```python
from build123d import *

# Parameters (mm, degrees)
AUFSATZ_LINEAR_START                        = 170
AUFSATZ_LINEAR_AUSTRAGEN2_DEPTH             = 460
SCHNITT_LINEAR_AUSTRAGEN1_REACH             = 14.65
SKIZZE15_R                                  = 4
SCHNITT_LINEAR_AUSTRAGEN1_DIRECTION_2_REACH = 14.65
SKIZZE17_W                                  = 30
SKIZZE17_H                                  = 20
SCHNITT_LINEAR_AUSTRAGEN2_DEPTH             = 12.65
SKIZZE19_W                                  = 17.7
SKIZZE19_H                                  = 170
SCHNITT_LINEAR_AUSTRAGEN3_DEPTH             = 25.15
HOLES_R                                     = 1.5
SCHNITT_LINEAR_AUSTRAGEN5_DEPTH             = 13.6500001
SCHNITT_LINEAR_AUSTRAGEN5_DEPTH_BACK        = 13.6500001
SKIZZE23_R                                  = 1.5
SCHNITT_LINEAR_AUSTRAGEN7_DEPTH             = 13.6500001
SCHNITT_LINEAR_AUSTRAGEN7_DEPTH_BACK        = 13.6500001


with BuildPart() as part:
    # Skizze10 (on Top Plane) → Aufsatz-Linear austragen2 (new body)
    with BuildSketch(Plane(origin=(0, 0, 0), x_dir=(1, 0, 0), z_dir=(0, 1, 0)).offset(AUFSATZ_LINEAR_START)):
        with BuildLine():
            Line((25.15, 12.65), (-12.6, 12.65))
            ThreePointArc((-12.6, 12.65), (-25.25, 0), (-12.6, -12.65))
            Line((-12.6, -12.65), (25.15, -12.65))
            Line((25.15, -12.65), (25.15, 12.65))
        make_face()
        with BuildLine():
            Line((23.35, 10.85), (-12.6, 10.85))
            ThreePointArc((-12.6, 10.85), (-23.45, 0), (-12.6, -10.85))
            Line((-12.6, -10.85), (23.35, -10.85))
            Line((23.35, -10.85), (23.35, 10.85))
        make_face(mode=Mode.SUBTRACT)
    extrude(amount=AUFSATZ_LINEAR_AUSTRAGEN2_DEPTH)

    # Schnitt-Linear austragen1: up to this face of the body (flat: up to its plane)
    schnitt_linear_austragen1_end = Plane(part.part.faces().sort_by_distance((6.275, 400, -12.65))[0])
    # Skizze15 → Schnitt-Linear austragen1 (cut, up to the picked face)
    with BuildSketch(Plane.XY, mode=Mode.PRIVATE) as schnitt_linear_austragen1_sk1:
        with Locations((-13.5, 190)):
            Circle(SKIZZE15_R)
    schnitt_linear_austragen1_tool1 = split(extrude(schnitt_linear_austragen1_sk1.sketch, amount=-SCHNITT_LINEAR_AUSTRAGEN1_REACH, mode=Mode.PRIVATE), bisect_by=schnitt_linear_austragen1_end, keep=Keep.BOTH, mode=Mode.PRIVATE)
    add(schnitt_linear_austragen1_tool1.solids().sort_by_distance((-13.5, 190, 0))[0], mode=Mode.SUBTRACT)
    # Skizze15 → Schnitt-Linear austragen1 (cut, up to the picked face)
    with BuildSketch(Plane.XY, mode=Mode.PRIVATE) as schnitt_linear_austragen1_sk2:
        with Locations((13.5, 190)):
            Circle(SKIZZE15_R)
    schnitt_linear_austragen1_tool2 = split(extrude(schnitt_linear_austragen1_sk2.sketch, amount=-SCHNITT_LINEAR_AUSTRAGEN1_REACH, mode=Mode.PRIVATE), bisect_by=schnitt_linear_austragen1_end, keep=Keep.BOTH, mode=Mode.PRIVATE)
    add(schnitt_linear_austragen1_tool2.solids().sort_by_distance((13.5, 190, 0))[0], mode=Mode.SUBTRACT)

    # Schnitt-Linear austragen1 direction 2: up to this face of the body (flat: up to its plane)
    schnitt_linear_austragen1_direction_2_end = Plane(part.part.faces().sort_by_distance((6.275, 400, 12.65))[0])
    # Skizze15 → Schnitt-Linear austragen1 direction 2 (cut, up to the picked face)
    with BuildSketch(Plane.XY, mode=Mode.PRIVATE) as schnitt_linear_austragen1_direction_2_sk1:
        with Locations((-13.5, 190)):
            Circle(SKIZZE15_R)
    schnitt_linear_austragen1_direction_2_tool1 = split(extrude(schnitt_linear_austragen1_direction_2_sk1.sketch, amount=SCHNITT_LINEAR_AUSTRAGEN1_DIRECTION_2_REACH, mode=Mode.PRIVATE), bisect_by=schnitt_linear_austragen1_direction_2_end, keep=Keep.BOTH, mode=Mode.PRIVATE)
    add(schnitt_linear_austragen1_direction_2_tool1.solids().sort_by_distance((-13.5, 190, 0))[0], mode=Mode.SUBTRACT)
    # Skizze15 → Schnitt-Linear austragen1 direction 2 (cut, up to the picked face)
    with BuildSketch(Plane.XY, mode=Mode.PRIVATE) as schnitt_linear_austragen1_direction_2_sk2:
        with Locations((13.5, 190)):
            Circle(SKIZZE15_R)
    schnitt_linear_austragen1_direction_2_tool2 = split(extrude(schnitt_linear_austragen1_direction_2_sk2.sketch, amount=SCHNITT_LINEAR_AUSTRAGEN1_DIRECTION_2_REACH, mode=Mode.PRIVATE), bisect_by=schnitt_linear_austragen1_direction_2_end, keep=Keep.BOTH, mode=Mode.PRIVATE)
    add(schnitt_linear_austragen1_direction_2_tool2.solids().sort_by_distance((13.5, 190, 0))[0], mode=Mode.SUBTRACT)

    # Skizze17 → Schnitt-Linear austragen2 (cut)
    with BuildSketch(Plane.XY):
        with Locations((1, 220)):
            Rectangle(SKIZZE17_W, SKIZZE17_H)
    extrude(amount=SCHNITT_LINEAR_AUSTRAGEN2_DEPTH, mode=Mode.SUBTRACT)

    # Skizze19 → Schnitt-Linear austragen3 (cut)
    with BuildSketch(Plane(origin=(0, 0, 0), x_dir=(0, 0, -1), z_dir=(1, 0, 0))):
        with Locations((0, 545)):
            Rectangle(SKIZZE19_W, SKIZZE19_H)
    extrude(amount=SCHNITT_LINEAR_AUSTRAGEN3_DEPTH, mode=Mode.SUBTRACT)

    # Holes → Schnitt-Linear austragen5 (cut, two sides)
    with BuildSketch(Plane.XY) as schnitt_linear_austragen5_sk:
        with Locations((18.35, 615)):
            Circle(HOLES_R)
        with Locations((-8, 615)):
            Circle(HOLES_R)
        with Locations((18.35, 234)):
            Circle(HOLES_R)
        with Locations((-8, 234)):
            Circle(HOLES_R)
    extrude(amount=SCHNITT_LINEAR_AUSTRAGEN5_DEPTH, mode=Mode.SUBTRACT)
    extrude(schnitt_linear_austragen5_sk.sketch, amount=-SCHNITT_LINEAR_AUSTRAGEN5_DEPTH_BACK, mode=Mode.SUBTRACT)

    # Skizze23 → Schnitt-Linear austragen7 (cut, two sides)
    with BuildSketch(Plane.XY) as schnitt_linear_austragen7_sk:
        with Locations((-8, 625)):
            Circle(SKIZZE23_R)
        with Locations((18.35, 625)):
            Circle(SKIZZE23_R)
    extrude(amount=SCHNITT_LINEAR_AUSTRAGEN7_DEPTH, mode=Mode.SUBTRACT)
    extrude(schnitt_linear_austragen7_sk.sketch, amount=-SCHNITT_LINEAR_AUSTRAGEN7_DEPTH_BACK, mode=Mode.SUBTRACT)


solid = part.part
```
Read the model definition and answer for the solid it produces. Units are mm, in the model's axes. A direction names the side the tool comes from. Coordinates: 2 decimals unless noted, no trailing zeros. Loops run counter-clockwise (first coordinate to the right, second up) from the corner with the lowest first, then second, coordinate; pieces in that order, holes last. Notation, with made-up numbers: (45, -29) - (97, -29) arc R27 ccw to (97, 0) - close; hole circle Ø9 at (60.5, -31). An arc over 180 degrees is marked (long way). Answer in a Markdown table with one row per item.
1. Find section C-C, the plane y = 302.5. Write down the section's boundary in (x, z), then the cut area to 3 significant figures.
Conclusion:
| item | result |
|---|---|
| outline | (-12.6, -12.65) - (25.15, -12.65) - (25.15, 12.65) - (-12.6, 12.65) arc R12.65 ccw to start; hole (-12.6, -10.85) - (23.35, -10.85) - (23.35, 10.85) - (-12.6, 10.85) arc R10.85 ccw to start |
| area | 241 mm² |
2. Find section B-B, the plane y = 527. Write down the section's boundary in (x, z), then the cut area to 3 significant figures.
Conclusion:
| item | result |
|---|---|
| outline | (-12.6, -12.65) - (25.15, -12.65) - (25.15, -8.85) - (23.35, -8.85) - (23.35, -10.85) - (-12.6, -10.85) arc R10.85 cw to (-12.6, 10.85) - (23.35, 10.85) - (23.35, 8.85) - (25.15, 8.85) - (25.15, 12.65) - (-12.6, 12.65) arc R12.65 ccw to start |
| area | 210 mm² |
3. Determine the mould class of faces 3 (the face through (7, 397, -12.65)), 4 (the face through (6, 397, -10.85)), 5 (the face through (-25.247, 396.78, -0.278)) for opening direction X: +X half, -X half, draft (parallel to the pull), parting line (faces both ways), or undercut.
Conclusion:
| item | result |
|---|---|
| face 3 | draft |
| face 4 | undercut |
| face 5 | -X half |
4. Given pin 1 (1.4 mm diameter, centred on x = 24.5, z = -2, fed in from +Y), flat-ended and moving along its own axis, determine where the tip first touches the part or whether it passes through.
Conclusion:
| item | result |
|---|---|
| pin 1 | stops at y = 460 |
5. Which of the six approach directions +Z, -Z, +X, -X, +Y, -Y give full straight-line access (tool end or side, diameter ignored) to faces 1 (the face through (5, 397, 10.85)), 2 (the face through (-2, 630, -11))?
Conclusion:
| item | result |
|---|---|
| face 1 | +Y, -Y |
| face 2 | +Z, -Z, +X, -X, +Y |
6. Find section A-A, the plane z = 0. Write down the section's boundary in (x, y).
Conclusion:
| item | result |
|---|---|
| outline | (-25.25, 170) - (-23.45, 170) - (-23.45, 630) - (-25.25, 630) - close; (23.35, 170) - (25.15, 170) - (25.15, 460) - (23.35, 460) - close |
7. Straight lines are drawn through the part: line 1 (Y direction, x = 18.35, z = 11.95); line 2 (X direction, y = 234, z = 11.7); line 3 (Z direction, x = 5.5, y = 605). For each, find the intervals that lie inside material, in ascending order.
Conclusion:
| item | result |
|---|---|
| line 1 | y = 170 to 232.5, 235.5 to 613.5, 616.5 to 623.5, 626.5 to 630 |
| line 2 | x = -17.41 to -9.5, -6.5 to 16.85, 19.85 to 25.15 |
| line 3 | z = -12.65 to -10.85, 10.85 to 12.65 |
